```python
from build123d import *

# Parameters (mm, degrees)
SKETCH1_W           = 312
SKETCH1_H           = 220
SKETCH1_R           = 3.5
SKETCH1_R_2         = 1
SKETCH1_W_2         = 13.4
SKETCH1_H_2         = 13.4
BOSS_EXTRUDE1_DEPTH = 10
FILLET1_R           = 5


with BuildPart() as part:
    # Sketch1 → Boss-Extrude1 (new body)
    with BuildSketch(Plane.XY):
        with Locations((156, 110)):
            Rectangle(SKETCH1_W, SKETCH1_H)
        with Locations((296, 212.7)):
            Circle(SKETCH1_R, mode=Mode.SUBTRACT)
        with Locations((287, 212.7)):
            Circle(SKETCH1_R_2, mode=Mode.SUBTRACT)
        with Locations((281, 212.7)):
            Circle(SKETCH1_R_2, mode=Mode.SUBTRACT)
        with Locations((148.6, 117.4)):
            Rectangle(SKETCH1_W_2, SKETCH1_H_2, mode=Mode.SUBTRACT)
        with Locations((163.4, 117.4)):
            Rectangle(SKETCH1_W_2, SKETCH1_H_2, mode=Mode.SUBTRACT)
        with Locations((148.6, 102.6)):
            Rectangle(SKETCH1_W_2, SKETCH1_H_2, mode=Mode.SUBTRACT)
        with Locations((163.4, 102.6)):
            Rectangle(SKETCH1_W_2, SKETCH1_H_2, mode=Mode.SUBTRACT)
    extrude(amount=BOSS_EXTRUDE1_DEPTH)

    # Fillet1
    fillet1_edges = [part.edges().sort_by_distance(p)[0] for p in [
        (0, 220, 5),
        (312, 220, 5),
        (312, 0, 5),
        (0, 0, 5),
    ]]
    fillet(fillet1_edges, radius=FILLET1_R)


solid = part.part
```
For this review, take the finished solid that the model builds, in its own axes (mm). A direction names the side the tool comes from. Round coordinates to 2 decimals unless told otherwise and drop trailing zeros. Write each loop counter-clockwise with the first axis right and the second up, starting at its lowest first coordinate (ties: lowest second). Pieces come first, ordered by that corner, then holes. Notation, with made-up numbers: (6, 23) -> (29, 23) arc R10 cw to (29, 34) -> close; hole circle Ø9 at (64.25, 60.25). An arc over 180 degrees is marked (long way). Use one line per item in the form item = value.
Q1. Consider section A-A (y = 103.5). State the section outline as (x, z) points, then the cut area to 3 significant figures.
Resolved:
outline = (0, 0) -> (141.9, 0) -> (141.9, 10) -> (0, 10) -> close; (155.3, 0) -> (156.7, 0) -> (156.7, 10) -> (155.3, 10) -> close; (170.1, 0) -> (312, 0) -> (312, 10) -> (170.1, 10) -> close
area = 2,850 mm²
Q2. Machinability: for faces 4 (the flat face through (154, 136, 10)), 5 (the flat face through (163, 110.7, 5)), which of the approach directions +Z, -Z, +X, -X, +Y, -Y give a long, thin tool a straight path to every point of the face, cutting with its end or side? Answer none if there is none.
Resolved:
face_4 = +Z, +X, -X, +Y, -Y
face_5 = +Z, -Z
Q3. The part is to be moulded in two halves that separate along Y. For faces 1 (the flat face through (154, 220, 5)), 2 (the flat face through (170.1, 103, 5)), 3 (the flat face through (0, 109, 5)), say which applies: released by +Y, released by -Y, zero draft, split by the parting line, or undercut.
Resolved:
face_1 = released by +Y
face_2 = undercut
face_3 = zero draft
Q4. To check wall thickness, follow probe 1 along X at (y, z) = (212.7, 2.75); probe 2 along X at (y, z) = (120.5, 2.75); probe 3 along Y at (x, z) = (296, 4.5). State the ranges of each line that lie inside material, in increasing order. Write a range as from..to.
Resolved:
probe_1 = 0..280, 282..286, 288..292.5, 299.5..312
probe_2 = 0..141.9, 155.3..156.7, 170.1..312
probe_3 = 0..209.2, 216.2..220
